from build123d import *

# Parameters (mm, degrees)
F0_W     = 25
F0_H     = 25
F1_DEPTH = 25
F2_T     = -2.5
F3_R     = 2.49999


# Not quite as in the source:
# - a fillet or chamfer is up to 0.001 mm smaller than in the source, because OpenCascade refuses the exact size


with BuildPart() as f1:
    # F0 (on Top) → F1 (new body)
    with BuildSketch(Plane.XY):
        with Locations((12.5, 12.5)):
            Rectangle(F0_W, F0_H)
    extrude(amount=F1_DEPTH)

    # F2
    f2_openings = [f1.faces().sort_by_distance(p)[0] for p in [
        (12.5, 0, 12.5),
    ]]
    offset(amount=F2_T, openings=f2_openings)

    # F3 (radius 2.5 in the source; OpenCascade refuses exactly that, so slightly less here)
    f3_edges = [f1.edges().sort_by_distance(p)[0] for p in [
        (12.5, 0, 25),
        (25, 12.5, 0),
        (12.5, 25, 0),
        (0, 12.5, 0),
        (25, 12.5, 25),
        (12.5, 25, 25),
        (0, 25, 12.5),
        (0, 0, 12.5),
        (0, 12.5, 25),
        (25, 0, 12.5),
        (25, 25, 12.5),
        (12.5, 0, 0),
    ]]
    fillet(f3_edges, radius=F3_R)


solid = f1.part
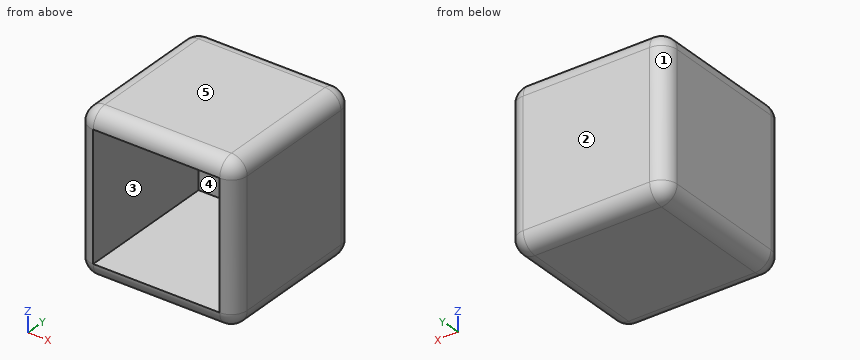
The listing builds one solid part. Answer for the finished solid, in the listing's coordinates (mm). Face numbers are marked on the shaded views. A direction names the side the tool comes from. Coordinates: 2 decimals unless noted, no trailing zeros. Order: outer loops, then holes, each group sorted by start corner. A loop starts at its lowest first (then second) coordinate and runs counter-clockwise, first axis right, second up.
Q1. Which of the six approach directions +Z, -Z, +X, -X, +Y, -Y give full straight-line access (tool end or side, diameter ignored) to the marked faces 4 and 5?
Q2. Consider line 1 (Z direction, x = 4.25, y = 6.5); line 2 (Y direction, x = 13.25, z = 12.25). Determine where each line is inside the solid, lowest interval first.
Q3. A cutting plane is placed at A-A, the plane y = 4. Write down the section's boundary in (x, z).
Q4. Given P1, Ø6, axis at x = 13.5, z = 17, coming from the -Y side, flat-ended and moving along its own axis, determine where the tip first touches the part or whether it passes through.
Q5. A cutting plane is placed at D-D, the plane z = 2. Write down the section's boundary in (x, y).
Q6. For a pull along X with two mould halves and no side action, classify the marked faces 1, 2 and 3 as pulls with the +X half, pulls with the -X half, needs draft (parallel to the pull), parting line crosses it, or undercut.
Answers follow:
1. face 4: -Y
1. face 5: +Z, +X, -X, +Y, -Y
2. line 1: z = 0 to 2.5, 22.5 to 25
2. line 2: y = 22.5 to 25
3. outline: (0, 2.5) arc R2.5 ccw to (2.5, 0) - (22.5, 0) arc R2.5 ccw to (25, 2.5) - (25, 22.5) arc R2.5 ccw to (22.5, 25) - (2.5, 25) arc R2.5 ccw to (0, 22.5) - close; hole (2.5, 2.5) - (22.5, 2.5) - (22.5, 22.5) - (2.5, 22.5) - close
4. P1: stops at y = 22.5
5. outline: (0.05, 2.5) arc R2.45 ccw to (2.5, 0.05) - (22.5, 0.05) arc R2.45 ccw to (24.95, 2.5) - (24.95, 22.5) arc R2.45 ccw to (22.5, 24.95) - (2.5, 24.95) arc R2.45 ccw to (0.05, 22.5) - close
6. face 1: pulls with the -X half
6. face 2: needs draft
6. face 3: undercut
